```python
from build123d import *

# Parameters (mm, degrees)
BOSS_EXTRUDE1_DEPTH = 4.5
SKETCH2_W           = 1
SKETCH2_H           = 11
BOSS_EXTRUDE2_DEPTH = 4.5
CUT_EXTRUDE1_DEPTH  = 51.20209159
CUT_EXTRUDE2_DEPTH  = 51.20209159
CUT_EXTRUDE3_DEPTH  = 51.20209159
SKETCH8_W           = 10
SKETCH8_H           = 4.5
BOSS_EXTRUDE3_DEPTH = 4.5
CUT_EXTRUDE4_DEPTH  = 34.948602328


with BuildPart() as part:
    # Sketch1 → Boss-Extrude1 (new body)
    with BuildSketch(Plane(origin=(0, 0, 0), x_dir=(0, 0, -1), z_dir=(1, 0, 0))):
        Polygon((0, 0), (0, -30), (-40, 0), align=None)
    extrude(amount=BOSS_EXTRUDE1_DEPTH)

    # Sketch2 → Boss-Extrude2 (add, through all)
    with BuildSketch(Plane(origin=(4.5, 0, 0), x_dir=(0, 0, -1), z_dir=(1, 0, 0))):
        with Locations((0.5, -20.25)):
            Rectangle(SKETCH2_W, SKETCH2_H)
    extrude(amount=-BOSS_EXTRUDE2_DEPTH)

    # Sketch3 → Cut-Extrude1 (cut, through all)
    with BuildSketch(Plane(origin=(4.5, 0, 0), x_dir=(0, 0, -1), z_dir=(1, 0, 0))):
        with BuildLine():
            Line((0, -4.45), (-4.5, -4.45))
            Line((-4.5, -4.45), (-4.5, -3.65))
            ThreePointArc((-4.5, -3.65), (-4.646446609, -3.296446609), (-5, -3.15))
            Line((-5, -3.15), (-7.5, -3.15))
            ThreePointArc((-7.5, -3.15), (-7.853553391, -3.296446609), (-8, -3.65))
            Line((-8, -3.65), (-8, -4.45))
            Line((-8, -4.45), (-11, -4.45))
            Line((-11, -4.45), (-11, -7.55))
            Line((-11, -7.55), (-8, -7.55))
            Line((-8, -7.55), (-8, -8.35))
            ThreePointArc((-8, -8.35), (-7.853553391, -8.703553391), (-7.5, -8.85))
            Line((-7.5, -8.85), (-5, -8.85))
            ThreePointArc((-5, -8.85), (-4.646446609, -8.703553391), (-4.5, -8.35))
            Line((-4.5, -8.35), (-4.5, -7.55))
            Line((-4.5, -7.55), (0, -7.55))
            Line((0, -7.55), (0, -4.45))
        make_face()
    extrude(amount=-CUT_EXTRUDE1_DEPTH, mode=Mode.SUBTRACT)

    # Sketch4 → Cut-Extrude2 (cut, through all)
    with BuildSketch(Plane(origin=(4.5, 0, 0), x_dir=(0, 0, -1), z_dir=(1, 0, 0))):
        with BuildLine():
            Line((-10.76, -21.93), (-13.24, -20.07))
            Line((-13.24, -20.07), (-10.54, -16.47))
            Line((-10.54, -16.47), (-11.18, -15.99))
            ThreePointArc((-11.18, -15.99), (-11.374974747, -15.660710678), (-11.28, -15.29))
            Line((-11.28, -15.29), (-9.78, -13.29))
            ThreePointArc((-9.78, -13.29), (-9.450710678, -13.095025253), (-9.08, -13.19))
            Line((-9.08, -13.19), (-8.44, -13.67))
            Line((-8.44, -13.67), (-6.64, -11.27))
            Line((-6.64, -11.27), (-4.16, -13.13))
            Line((-4.16, -13.13), (-5.96, -15.53))
            Line((-5.96, -15.53), (-5.32, -16.01))
            ThreePointArc((-5.32, -16.01), (-5.125025253, -16.339289322), (-5.22, -16.71))
            Line((-5.22, -16.71), (-6.72, -18.71))
            ThreePointArc((-6.72, -18.71), (-7.049289322, -18.904974747), (-7.42, -18.81))
            Line((-7.42, -18.81), (-8.06, -18.33))
            Line((-8.06, -18.33), (-10.76, -21.93))
        make_face()
    extrude(amount=-CUT_EXTRUDE2_DEPTH, mode=Mode.SUBTRACT)

    # Sketch5 → Cut-Extrude3 (cut, through all)
    with BuildSketch(Plane(origin=(4.5, 0, 0), x_dir=(0, 0, -1), z_dir=(1, 0, 0))):
        Polygon((-15.24, -18.57), (-15.24, 0), (-40, 0), align=None)
    extrude(amount=-CUT_EXTRUDE3_DEPTH, mode=Mode.SUBTRACT)

    # Sketch8 → Boss-Extrude3 (add, through all)
    with BuildSketch(Plane(origin=(4.5, 0, 0), x_dir=(0, 0, -1), z_dir=(1, 0, 0))):
        with Locations((-10, 2.25)):
            Rectangle(SKETCH8_W, SKETCH8_H)
    extrude(amount=-BOSS_EXTRUDE3_DEPTH)

    # Sketch10 → Cut-Extrude4 (cut, through all)
    with BuildSketch(Plane(origin=(4.5, 0, 0), x_dir=(0, 0, -1), z_dir=(1, 0, 0))):
        Polygon((0, -28.25), (-2.333333333, -28.25), (0, -30), align=None)
    extrude(amount=-CUT_EXTRUDE4_DEPTH, mode=Mode.SUBTRACT)


solid = part.part
```
The listing builds one solid part. Answer for the finished solid, in the listing's coordinates (mm). A direction names the side the tool comes from. Round coordinates to 2 decimals unless told otherwise and drop trailing zeros. Loops run counter-clockwise (first coordinate to the right, second up) from the corner with the lowest first, then second, coordinate; pieces in that order, holes last.
1) For faces 1 (the face through (4.5, -12, 9)), 2 (the face through (2, 2, 15)), 3 (the face through (2, -4.45, 9)), 4 (the face through (2, -4, 8)), 5 (the face through (2, -11, 0)), determine the directions among +Z, -Z, +X, -X, +Y, -Y from which every point of the face is accessible in a straight line to the end or side of a thin tool.
Outcome:
face 1: +Z, -Z, +X, +Y, -Y
face 2: +Z, +X, -X, +Y
face 3: -Z, +X, -X
face 4: +X, -X
face 5: -Z, +X, -X, +Y
2) Given P1, Ø1.3, axis at x = 3, y = 1.5, coming from the +Z side; P2, Ø2, axis at x = 3, y = 1.5, coming from the -Z side; P3, Ø0.5, axis at x = 2.5, z = -0.5, coming from the -Y side, each flat-ended and moving along its own axis, determine where each tip first touches the part or whether it passes through.
Outcome:
P1: stops at z = 15
P2: stops at z = 5
P3: stops at y = -25.75
3) Consider line 1 (Y direction, x = 3.45, z = 9); line 2 (Z direction, x = 4.25, y = -18.5); line 3 (Y direction, x = 0.9, z = 6.25). Determine where each line is inside the solid, lowest interval first.
Outcome:
line 1: y = -23.25 to -19.58, -13.25 to -7.55, -4.45 to 4.5
line 2: z = -1 to 6.56, 7.83 to 8.19, 12.06 to 15.24
line 3: y = -25.31 to -18.08, -11.56 to -8.85, -3.15 to 4.5
4) A cutting plane is placed at B-B on z = 8.75. Determine the outline of the cut face in (x, y).
Outcome:
outline: (0, -23.44) - (4.5, -23.44) - (4.5, -19.25) - (0, -19.25) - close; (0, -13.44) - (4.5, -13.44) - (4.5, -7.55) - (0, -7.55) - close; (0, -4.45) - (4.5, -4.45) - (4.5, 4.5) - (0, 4.5) - close
5) For a pull along Y with two mould halves and no side action, classify faces 6 (the face through (2.3, -14.75, -0.5)), 7 (the face through (2, -8.85, 6)), 8 (the face through (2, -28.25, 1)) as released by +Y, released by -Y, zero draft, split by the parting line, or undercut.
Outcome:
face 6: released by +Y
face 7: undercut
face 8: released by -Y
6) A cutting plane is placed at A-A on z = 1.25. Determine the outline of the cut face in (x, y), plus the area to 3 significant figures.
Outcome:
outline: (0, -28.25) - (4.5, -28.25) - (4.5, -7.55) - (0, -7.55) - close; (0, -4.45) - (4.5, -4.45) - (4.5, 0) - (0, 0) - close
area: 113 mm2
7) A cutting plane is placed at D-D on z = 3. Determine the outline of the cut face in (x, y).
Outcome:
outline: (0, -27.75) - (4.5, -27.75) - (4.5, -7.55) - (0, -7.55) - close; (0, -4.45) - (4.5, -4.45) - (4.5, 0) - (0, 0) - close
8) A cutting plane is placed at C-C on y = -2.5. Determine the outline of the cut face in (x, z).
Outcome:
outline: (0, 0) - (4.5, 0) - (4.5, 15.24) - (0, 15.24) - close
